Could you check a few things on this model? Use its own coordinates, in mm. A direction names the side the tool comes from. Give positions to 0.01 mm unless a question says otherwise; leave off trailing zeros. Loops run counter-clockwise (first coordinate to the right, second up) from the corner with the lowest first, then second, coordinate; pieces in that order, holes last. Notation, with made-up numbers: (55, -37.5) -> (109, -37.5) arc R19 cw to (109, -24.5) -> close; hole circle Ø1 at (-23.5, 59). An arc over 180 degrees is marked (long way). Put each result on its own line as item: value.
```python
from build123d import *

# Parameters (mm, degrees)
BOSS_EXTRUDE1_DEPTH = 48
CUT_EXTRUDE1_DEPTH  = 110.494292089


with BuildPart() as part:
    # Sketch2 → Boss-Extrude1 (new body)
    with BuildSketch(Plane.XY):
        Polygon((0, 0), (0, 46), (-47, 46), (-87, 10), (-87, 0), align=None)
    extrude(amount=BOSS_EXTRUDE1_DEPTH)

    # Sketch3 → Cut-Extrude1 (cut, through all)
    with BuildSketch(Plane(origin=(0, 0, 0), x_dir=(0, 0, -1), z_dir=(1, 0, 0))):
        Polygon((-28, 46), (-20, 46), (-20, 31), (-10, 31), (-10, 16), (-38, 16), (-38, 31), (-28, 31), align=None)
    extrude(amount=-CUT_EXTRUDE1_DEPTH, mode=Mode.SUBTRACT)


solid = part.part
```
1. I need wall thicknesses on line 1 (Z direction, x = -14, y = 22); line 2 (Y direction, x = -23, z = 17.5); line 3 (Z direction, x = -32, y = 43). Which ranges of each line are inside material? Lowest first, please.
Recorded:
line 1: z = 0 to 10, 38 to 48
line 2: y = 0 to 16, 31 to 46
line 3: z = 0 to 20, 28 to 48
2. If we section it at C-C (x = -62): List the corners of the cut face in (y, z) for me.
Recorded:
outline: (0, 0) -> (32.5, 0) -> (32.5, 20) -> (31, 20) -> (31, 10) -> (16, 10) -> (16, 38) -> (31, 38) -> (31, 28) -> (32.5, 28) -> (32.5, 48) -> (0, 48) -> close
3. If we section it at D-D (y = 18.5): List the corners of the cut face in (x, z) for me, then the cut area to 3 significant figures.
Recorded:
outline: (-77.56, 0) -> (0, 0) -> (0, 10) -> (-77.56, 10) -> close; (-77.56, 38) -> (0, 38) -> (0, 48) -> (-77.56, 48) -> close
area: 1,550 mm^2
4. Thinking about a two-plate mould opening in Y: for faces 4 (the face through (-23, 46, 38)), 5 (the face through (-40, 24, 10)), 6 (the face through (-34, 23, 0)), which applies, pulls with the +Y half, pulls with the -Y half, needs draft (parallel to the pull), parting line crosses it, or undercut?
Recorded:
face 4: pulls with the +Y half
face 5: undercut
face 6: needs draft
5. If we section it at B-B (y = 28): List the corners of the cut face in (x, z) for me.
Recorded:
outline: (-67, 0) -> (0, 0) -> (0, 10) -> (-67, 10) -> close; (-67, 38) -> (0, 38) -> (0, 48) -> (-67, 48) -> close
6. If we section it at A-A (z = 31.5): List the corners of the cut face in (x, y) for me, then the cut area to 3 significant figures.
Recorded:
outline: (-87, 0) -> (0, 0) -> (0, 16) -> (-80.33, 16) -> (-87, 10) -> close; (-63.67, 31) -> (0, 31) -> (0, 46) -> (-47, 46) -> close
area: 2,200 mm^2
7. For faces 1 (the face through (-31, 31, 33)), 2 (the face through (-24, 38, 28)), 3 (the face through (-62.28, 32.25, 18.33)), which set-ups out of +Z, -Z, +X, -X, +Y, -Y let a thin tool reach every point of the face, with its end or its side?
Recorded:
face 1: +X, -X
face 2: +X, -X, +Y
face 3: +Z, -Z, -X, +Y
8. I'm going to push flat-ended pins straight in: pin 1 (8.5 mm diameter, centred on x = -52.5, z = 30, fed in from +Y) (3 decimals); pin 2 (4 mm diameter, centred on y = 13, z = 19, fed in from -X). Where does each tip first touch, or does it pass through?
Recorded:
pin 1: stops at y = 44.875
pin 2: stops at x = -85.89
